Job drawing, mm, ordinate dimensions from the low corner. One solid piece. Give positions to 0.01 mm unless a question says otherwise; leave off trailing zeros. Loops run counter-clockwise (first coordinate to the right, second up) from the corner with the lowest first, then second, coordinate; pieces in that order, holes last. Notation, with made-up numbers: M 53,12.25 L 65,12.25 A8 ccw 65,27.25 Z; hole C 19,-13 d1. An arc over 180 degrees is marked long. Answer in a Markdown table with one row per item.
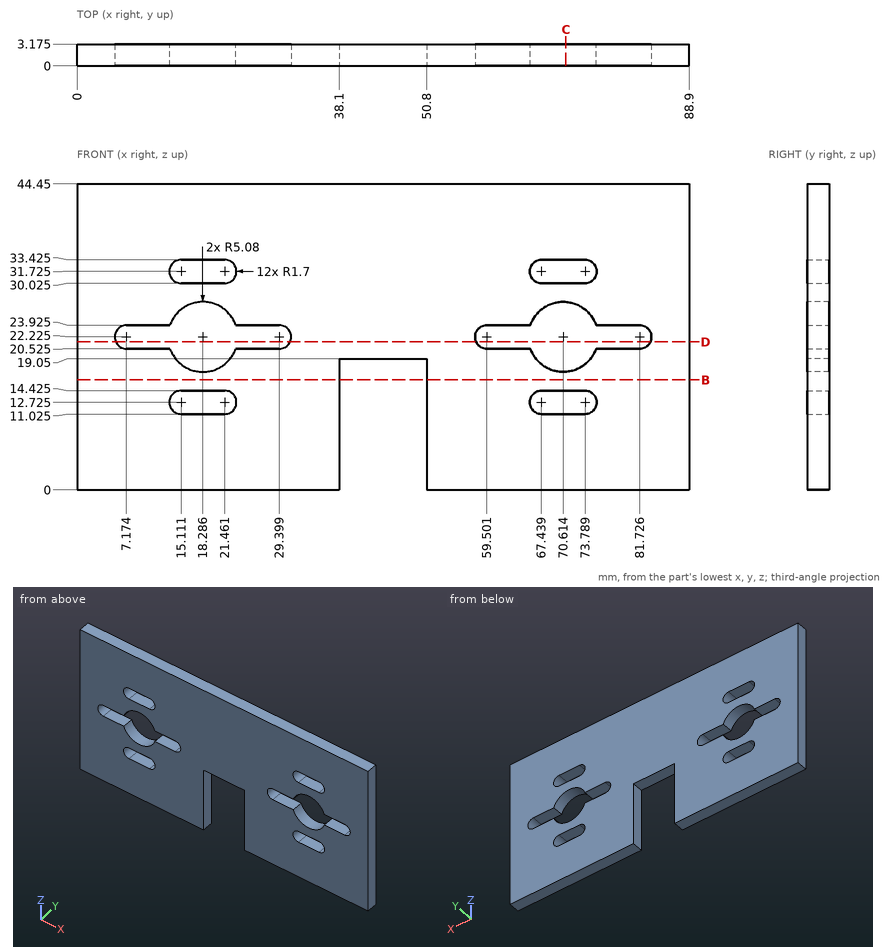
(1) Pin check, flat tip, straight feed: pin 1 Ø1.6 at (x, y) = (18.5, 2) entering from -Z. Stop position of the tip, or through.
Recorded:
| item | result |
|---|---|
| pin 1 | stops at z = 0 |
(2) Saw through at C-C (x = 71). Give the number of separate pieces and of enclosed holes in the cut face.
Recorded:
| item | result |
|---|---|
| separate pieces | 4 |
| enclosed holes | 0 |
(3) Saw through at D-D (z = 21.5). Write the cut outline in (x, y) (1 decimal), plus the area to 3 significant figures.
Recorded:
| item | result |
|---|---|
| outline | M 0,0 L 5.6,0 L 5.6,3.2 L 0,3.2 Z; M 30.9,0 L 58,0 L 58,3.2 L 30.9,3.2 Z; M 83.3,0 L 88.9,0 L 88.9,3.2 L 83.3,3.2 Z |
| area | 122 mm^2 |
(4) Drill centre lines: line 1 along X through (y, z) = (0.2, 16); line 2 along X through (y, z) = (2.15, 23); line 3 along X through (y, z) = (1.95, 13). Where is each one in solid material? Low to high.
Recorded:
| item | result |
|---|---|
| line 1 | x = 0 to 38.1, 50.8 to 88.9 |
| line 2 | x = 0 to 5.66, 30.91 to 57.99, 83.24 to 88.9 |
| line 3 | x = 0 to 13.43, 23.14 to 38.1, 50.8 to 65.76, 75.47 to 88.9 |
(5) Saw through at B-B (z = 16). Write the cut outline in (x, y) (1 decimal), plus the area to 3 significant figures.
Recorded:
| item | result |
|---|---|
| outline | M 0,0 L 38.1,0 L 38.1,3.2 L 0,3.2 Z; M 50.8,0 L 88.9,0 L 88.9,3.2 L 50.8,3.2 Z |
| area | 242 mm^2 |
